```python
from build123d import *

# Parameters (mm, degrees)
SKETCH2_R               = 19
BASENUT_DEPTH           = 9.1
CHAMFER1_SIZE           = 0.5
SKETCH3_R               = 11.188
HOLE_DEPTH              = 10.1
ENDCHAMFER_SIZE2        = 0.5
ENDCHAMFER_SIZE         = 0.866025404
ENDCHAMFER_EDGE_2_SIZE2 = 0.5
ENDCHAMFER_EDGE_2_SIZE  = 0.866025404
SLOTCUT_DEPTH           = 10.1
SLOTPAT_COUNT           = 4
LPATTERN10_COUNT        = 8
LPATTERN10_PITCH        = 0.9744


with BuildPart() as part:
    # Sketch2 → BaseNut (new body)
    with BuildSketch(Plane.XY):
        Circle(SKETCH2_R)
    extrude(amount=-BASENUT_DEPTH)

    # Chamfer1
    chamfer1_edges = [part.edges().sort_by_distance(p)[0] for p in [
        (-19, 0, 0),
        (-19, 0, -9.1),
    ]]
    chamfer(chamfer1_edges, length=CHAMFER1_SIZE)

    # Sketch3 → Hole (cut, through all)
    with BuildSketch(Plane(origin=(-17.561722019, 31.682666601, 0), x_dir=(1, 0, 0), z_dir=(0, 0, 1))):
        with Locations((17.561722019, -31.682666601)):
            Circle(SKETCH3_R)
    extrude(amount=-HOLE_DEPTH, mode=Mode.SUBTRACT)

    # EndChamfer
    endchamfer_edges = [part.edges().sort_by_distance(p)[0] for p in [
        (-11.188, 0, -9.1),
    ]]
    chamfer(endchamfer_edges, length=ENDCHAMFER_SIZE, length2=ENDCHAMFER_SIZE2)

    # EndChamfer edge 2
    endchamfer_edge_2_edges = [part.edges().sort_by_distance(p)[0] for p in [
        (-11.188, 0, 0),
    ]]
    chamfer(endchamfer_edge_2_edges, length=ENDCHAMFER_EDGE_2_SIZE, length2=ENDCHAMFER_EDGE_2_SIZE2)

    # Sketch4 → SlotCut (cut, through all)
    with BuildSketch(Plane(origin=(-28.84840977, 49.266341409, 0), x_dir=(1, 0, 0), z_dir=(0, 0, 1))):
        with BuildLine():
            Line((26.34840977, -30.431533207), (26.34840977, -32.431533207))
            Line((26.34840977, -32.431533207), (31.34840977, -32.431533207))
            Line((31.34840977, -32.431533207), (31.34840977, -30.431533207))
            ThreePointArc((31.34840977, -30.431533207), (28.84840977, -30.266341409), (26.34840977, -30.431533207))
        make_face()
    slotcut = extrude(amount=-SLOTCUT_DEPTH, mode=Mode.SUBTRACT)

    # SlotPat: SlotCut ×4 about axis
    slotpat_axis = Axis((0, 0, 0), (0, 0, 1))
    for i in range(1, SLOTPAT_COUNT):
        add(slotcut.rotate(slotpat_axis, i * 360 / SLOTPAT_COUNT), mode=Mode.SUBTRACT)

    # Sketch5 → Cut-Revolve10 (revolve, cut)
    with BuildSketch(Plane(origin=(0, 0, 0), x_dir=(1, 0, 0), z_dir=(0, 1, 0))):
        Polygon((10.376, 1.272025404), (10.376, 0.460025404), (11.188, 0.460025404), (11.891212628, 0.866025404), (11.188, 1.272025404), align=None)
    cut_revolve10 = revolve(axis=Axis((0, 0, -37.301805437), (0, 0, 1)), mode=Mode.SUBTRACT)

    # LPattern10: Cut-Revolve10 ×8
    with Locations(*[(0, 0, -i * LPATTERN10_PITCH) for i in range(1, LPATTERN10_COUNT)]):
        add(cut_revolve10, mode=Mode.SUBTRACT)


solid = part.part
```
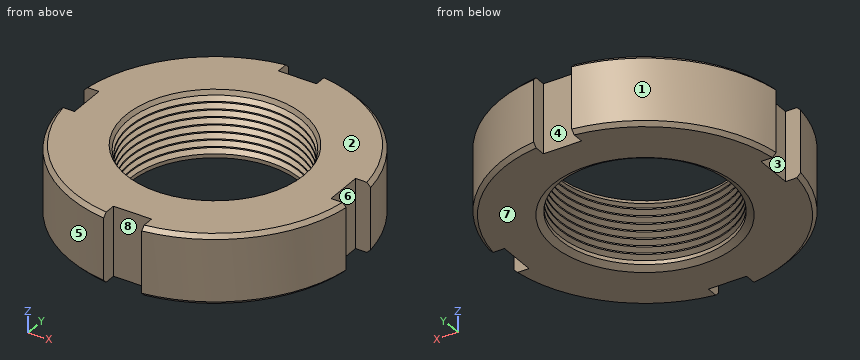
Input: part model. Units: mm. Frame: model coordinates. Face numbers are marked on the shaded views. A direction names the side the tool comes from. Coordinates: 2 decimals unless noted, no trailing zeros. One line per item, written item: value.
(1) Pin query (flat end, axial travel): pin 1 (0.6 mm diameter, centred on y = 17.5, z = -6, fed in from -X); pin 2 (1.5 mm diameter, centred on x = 7.5, z = -4.5, fed in from +Y); pin 3 (4 mm diameter, centred on y = 0, z = -6, fed in from +X). Return the tip coordinate at first contact, or that it passes through.
Filled in:
pin 1: x = -8.07
pin 2: y = 17.76
pin 3: x = 16.83
(2) Line query: line 1 along Y through (x, z) = (0, -7.2); line 2 along X through (y, z) = (-10, -0.5); line 3 along X through (y, z) = (4.5, -5). Output: solid intervals per line, ascending. Write a range as from..to.
Filled in:
line 1: -16.83..-11.19, 11.19..16.83
line 2: -16.16..-5.47, 5.47..16.16
line 3: -18.46..-10.56, 10.56..18.46
(3) Reachability of the marked faces 4, 5, 6, 7 and 8 from +Z, -Z, +X, -X, +Y, -Y: full face, straight path, thin tool, end or side. Return the list, or none.
Filled in:
face 4: +Z, -Z, +Y
face 5: +Z, -Z, -X, -Y
face 6: +Z, -Z, +X
face 7: -Z, +X, -X, +Y, -Y
face 8: +Z, -Z, -Y
(4) Pull-direction query (Y, two-part tool) for the marked faces 1, 2 and 3; classes: +Y half, -Y half, draft (parallel to the pull), parting line (faces both ways), or undercut.
Filled in:
face 1: +Y half
face 2: draft
face 3: undercut
